Autodesk Inventor part; units mm, degrees
ref_plane "Work Plane2" through (0, -4.8088, -18.4315) normal (-1, 0, 0) x (0, 0, 1)
ref_plane "YZ Plane" through (0, 0, 0) normal (1, 0, 0) x (0, 1, 0)
ref_plane "XZ Plane" through (0, 0, 0) normal (0, 1, 0) x (-1, 0, 0)
ref_plane "Work Plane1" through (5, 13.3547, -3.0565) normal (1, 0, 0) x (0, -1, 0)
ref_plane "Work Plane2" through (0, -4.8088, -18.4315) normal (-1, 0, 0) x (0, 0, 1)
sketch "Sketch1" plane through (5, 13.3547, -3.0565) normal (1, 0, 0) x (0, -1, 0)
  arc A0 (6.1228, -3.0565) -> (-6.1228, -3.0565) centre (0, 0) ccw
  line L0 (6.1228, -3.0565) -> (18.1635, -3.0565)
  line L1 (18.1635, -3.0565) -> (18.1635, 15.375)
  line L2 (18.1635, 15.375) -> (-18.375, 15.375)
  line L3 (-18.375, 15.375) -> (-18.375, -3.0565)
  line L4 (-18.375, -3.0565) -> (-6.1228, -3.0565)
  circle A1 centre (8, 0) radius 1.0564
  circle A2 centre (-8, 0) radius 1.0564
  circle A3 centre (8, 0) radius 1.0564
  circle A4 centre (-8, 0) radius 1.0564
  circle A5 centre (0, 0) radius 5
  circle A6 centre (0, 0) radius 13.7
  line L5 (18.1635, 15.375) -> (18.1635, 1)
  line L6 (18.1635, 1) -> (13.6635, 1)
  arc A7 (13.6635, 1) -> (-13.6635, 1) centre (0, 0) ccw
  line L7 (-13.6635, 1) -> (-18.375, 1)
  line L8 (-18.375, 1) -> (-18.375, -15.125)
  line L9 (55.7975, -15.125) -> (-18.375, -15.125)
  line L10 (55.7975, -15.125) -> (55.7975, 5.375)
  line L11 (55.7975, 5.375) -> (48.7975, 5.375)
  line L12 (48.7975, 5.375) -> (48.7975, 15.375)
  line L13 (48.7975, 15.375) -> (18.1635, 15.375)
  line L14 (-18.375, -15.125) -> (18.1635, -15.125)
  line L15 (18.1635, -15.125) -> (18.1635, -5.0565)
  line L16 (18.1635, -5.0565) -> (-18.375, -5.0565)
  line L17 (-18.375, -5.0565) -> (-18.375, -15.125)
  circle A8 centre (0, 0) radius 9
  point P0 (13.3547, -3.0565)
  point P1 (7.4453, -5.0565)
  point P2 (-7.4453, -5.0565)
  point P3 (-18.375, -5.0565)
  point P4 (18.1635, -15.125)
  point P5 (12.7327, -5.0565)
  point P6 (-12.7327, -5.0565)
  dimension "d0" = 2
  dimension "d1" = 18
extrude "Extrusion1" add sketch "Sketch1" against normal up to surface (5 mm away) contours L16 L15 L9 L8 A6
sketch "Sketch2" plane through (5, -4.8088, 12.0685) normal (0, 0, 1) x (1, 0, 0)
  line L0 (-5, 4.8088) -> (0, 4.8088)
  line L1 (-5, 4.8088) -> (-5, 0)
  line L2 (-5, 0) -> (4.7, 0)
  line L3 (4.7, 12.0407) -> (4.7, 0)
  line L4 (0, 12.0407) -> (4.7, 12.0407)
  line L5 (0, 12.0407) -> (0, 4.8088)
  line L6 (-5, 36.5385) -> (4.7, 36.5385)
  line L7 (-5, 36.5385) -> (-5, 31.5181)
  line L8 (-5, 31.5181) -> (0, 31.5181)
  line L9 (0, 31.5181) -> (0, 24.2862)
  line L10 (0, 24.2862) -> (4.7, 24.2862)
  line L11 (4.7, 36.5385) -> (4.7, 24.2862)
  point P0 (-2, 2.2)
  point P1 (-2, 34.3385)
  dimension "d6" = 2.2
  dimension "d7" = 2.2
  dimension "d8" = 3
  dimension "d9" = 3
hole "Hole1" at (3, -2.6088, 12.0685) at (3, 29.5297, 12.0685) direction (0, 0, -1) diameter 3.6 end through all countersink diameter 6.5 countersink angle 90
properties part number "right_motor_ceil_2"
Read the model definition and answer for the solid it produces. Units are mm, in the model's axes. Round coordinates to 2 decimals unless told otherwise and drop trailing zeros. Order: outer loops, then holes, each group sorted by start corner. A loop starts at its lowest first (then second) coordinate and runs counter-clockwise, first axis right, second up.
1) The mould has two halves that part along X. Classify faces 1 (the face through (1.75, -0.98, 10.87)), 2 (the face through (2.54, 13.58, 10.64)), 3 (the face through (0, 14, 11)): released by +X, released by -X, zero draft, split by the parting line, or undercut.
2) The part is cut by section A-A on z = 6. Write down the section's boundary in (x, y).
3) The part is cut by section C-C on z = 8.25. Write down the section's boundary in (x, y).
4) The part is cut by section D-D on y = 16. Write down the section's boundary in (x, z).
5) The part is cut by section B-B on x = 3. Write down the section's boundary in (y, z), plus the area to 3 significant figures.
6) A flat-ended cylindrical pin translates along its axis: pin 1 (1 mm diameter, centred on y = 17, z = 9.5, fed in from -X). Find the tip coordinate at first contact, or state that the pin passes through.
7) Straight lines are drawn through the part: L1, parallel to Y at x = 4.05, z = 11; L2, parallel to Y at x = 2, z = 4.5; L3, parallel to Y at x = 3, z = 6.25. For each, find the intervals that lie inside material, in ascending order.
Resolved:
1. face 1: undercut
1. face 2: zero draft
1. face 3: released by -X
2. outline: (0, -4.81) - (5, -4.81) - (5, 3.08) - (0, 3.08) - close; (0, 23.63) - (5, 23.63) - (5, 31.73) - (0, 31.73) - close; hole circle Ø3.6 at (3, -2.61); hole circle Ø3.6 at (3, 29.53)
3. outline: (0, -4.81) - (5, -4.81) - (5, 5.62) - (0, 5.62) - close; (0, 21.09) - (5, 21.09) - (5, 31.73) - (0, 31.73) - close; hole circle Ø3.6 at (3, -2.61); hole circle Ø3.6 at (3, 29.53)
4. outline: (0, 10.39) - (5, 10.39) - (5, 12.07) - (0, 12.07) - close
5. outline: (-4.81, 2) - (-4.41, 2) - (-4.41, 10.62) - (-4.81, 11.02) - close; (-0.81, 2) - (0.62, 2) arc R13.7 cw to (26.09, 2) - (27.73, 2) - (27.73, 10.62) - (26.28, 12.07) - (0.64, 12.07) - (-0.81, 10.62) - close; (31.33, 2) - (31.73, 2) - (31.73, 11.02) - (31.33, 10.62) - close
5. area: 133 mm2
6. pin 1: passes through
7. L1: y = -4.81 to -4.52, -0.7 to 27.62, 31.44 to 31.73
7. L2: y = -4.81 to -4.11, -1.11 to 1.93, 24.78 to 28.03, 31.03 to 31.73
7. L3: y = -4.81 to -4.41, -0.81 to 3.3, 23.41 to 27.73, 31.33 to 31.73
